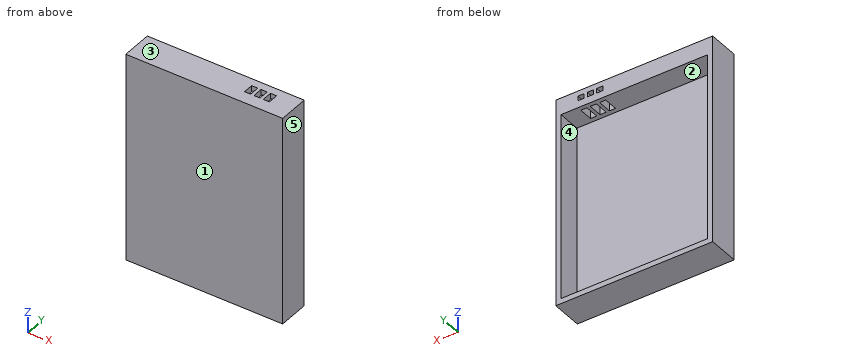
Autodesk Inventor part; units mm, degrees
ref_plane "YZ Plane" through (0, 0, 0) normal (1, 0, 0) x (0, 1, 0)
ref_plane "XZ Plane" through (0, 0, 0) normal (0, 1, 0) x (-1, 0, 0)
ref_plane "XY Plane" through (0, 0, 0) normal (0, 0, 1) x (1, 0, 0)
sketch "Sketch2" plane through (0, 0, 0) normal (0, 1, 0) x (-1, 0, 0)
  line L0 (11.0925, -17.7456) -> (-22.3075, -17.7456)
  line L1 (-22.3075, -17.7456) -> (-22.3075, 24.2544)
  line L2 (-22.3075, 24.2544) -> (11.0925, 24.2544)
  line L3 (11.0925, 24.2544) -> (11.0925, -17.7456)
  point P0 (0, 0)
  dimension "d2" = 42
  dimension "d3" = 33.4
extrude "Extrusion1" add sketch "Sketch2" along normal blind 6
sketch "Sketch3" plane through (0, 6, 0) normal (0, 1, 0) x (1, 0, 0)
  line L0 (-9.9925, 16.6456) -> (21.2075, 16.6456)
  line L1 (21.2075, 16.6456) -> (21.2075, -23.1544)
  line L2 (21.2075, -23.1544) -> (-9.9925, -23.1544)
  line L3 (-9.9925, -23.1544) -> (-9.9925, 16.6456)
  line L4 (22.3075, 17.7456) -> (-11.0925, 17.7456)
  line L5 (-11.0925, 17.7456) -> (-11.0925, -24.2544)
  line L6 (22.3075, -24.2544) -> (22.3075, 17.7456)
  line L7 (-11.0925, -24.2544) -> (22.3075, -24.2544)
  point P0 (0, 0)
  dimension "d6" = 1.1
  dimension "d7" = 1.1
  dimension "d8" = 1.1
  dimension "d9" = 1.1
  dimension "d10" = 39.8
extrude "Extrusion2" cut sketch "Sketch3" against normal blind 4.9 contours L0 L1 L2 L3
sketch "Sketch4" plane through (0, 0, 0) normal (0, -1, 0) x (1, 0, 0)
  line L0 (22.3075, -17.7456) -> (-11.0925, -17.7456)
  line L1 (-11.0925, -17.7456) -> (-11.0925, 24.2544)
  line L2 (22.3075, -17.7456) -> (-11.0925, -17.7456)
  line L3 (-11.0925, -17.7456) -> (-11.0925, 24.2544)
  line L4 (-11.0925, 24.2544) -> (22.3075, 24.2544)
  line L5 (22.3075, 24.2544) -> (22.3075, -17.7456)
  point P0 (0, 0)
extrude "Extrusion3" add sketch "Sketch4" along normal blind 0.6
sketch "Sketch5" plane through (-11.0925, 6, 24.2544) normal (0, 0, 1) x (1, 0, 0)
  line L0 (33.4, -6.6) -> (33.4, 0)
  line L1 (33.4, -6.6) -> (0, -6.6)
  line L2 (0, -6.6) -> (0, -2.5)
  line L3 (0, -2.5) -> (33.4, -2.5)
  line L4 (33.4, -2.5) -> (33.4, -6.6)
  point P0 (11.0925, -6)
  point P1 (33.4, -2.5)
extrude "Extrusion4" add sketch "Sketch5" along normal blind 3
sketch "Sketch6" plane through (21.2075, 6, 23.1544) normal (0, 0, -1) x (-1, 0, 0)
  line L0 (3.6, -0.9) -> (4.9, -0.9)
  line L1 (4.9, -0.9) -> (4.9, -3.9)
  line L2 (4.9, -3.9) -> (3.6, -3.9)
  line L3 (3.6, -3.9) -> (3.6, -0.9)
  line L4 (0, -4.9) -> (31.2, -4.9)
  line L5 (5.6, -0.9) -> (6.9, -0.9)
  line L6 (6.9, -0.9) -> (6.9, -3.9)
  line L7 (6.9, -3.9) -> (5.6, -3.9)
  line L8 (5.6, -3.9) -> (5.6, -0.9)
  line L9 (7.6, -0.9) -> (8.9, -0.9)
  line L10 (8.9, -0.9) -> (8.9, -3.9)
  line L11 (8.9, -3.9) -> (7.6, -3.9)
  line L12 (7.6, -3.9) -> (7.6, -0.9)
  point P0 (21.2075, -6)
  point P1 (0, 0)
  dimension "d17" = 3
  dimension "d18" = 1.3
  dimension "d19" = 3.6
  dimension "d20" = 1
  dimension "d23" = 3
  dimension "d24" = 1.3
  dimension "d25" = 3
  dimension "d26" = 1.3
  dimension "d27" = 1
  dimension "d28" = 1
  dimension "d29" = 0.7
  dimension "d30" = 0.7
sketch "Sketch7" plane through (-11.0925, 3.5, 24.2544) normal (0, 1, 0) x (1, 0, 0)
  line L0 (0, 0) -> (33.4, 0)
  line L1 (0, 42) -> (0, -3)
  line L2 (33.4, 0) -> (0, 0)
  line L3 (0, 0) -> (0, -3)
  line L4 (0, -3) -> (33.4, -3)
  line L5 (33.4, -3) -> (33.4, 0)
  point P0 (11.0925, 24.2544)
extrude "Extrusion5" add sketch "Sketch7" along normal blind 2.5
extrude "Extrusion6" cut sketch "Sketch6" against normal through all
sketch "Sketch8" plane through (0, 6, 0) normal (0, 1, 0) x (1, 0, 0)
  point P0 (0, 0)
sketch "Sketch9" plane through (16.3075, 2.1, 23.1544) normal (0, 1, 0) x (1, 0, 0)
  line L0 (1.3, 0) -> (1.3, -4.1)
  line L1 (0, 0) -> (0, -4.1)
  line L2 (1.3, -2.3) -> (0, -2.3)
  line L3 (0, -2.3) -> (0, -2)
  line L4 (0, -2) -> (1.3, -2)
  line L5 (1.3, -2) -> (1.3, -2.3)
  line L6 (0, 0) -> (1.3, 0)
  line L7 (-0.7, -2.3111) -> (-2, -2.3111)
  line L8 (-2, -2.3111) -> (-2, -2.0111)
  line L9 (-2, -2.0111) -> (-0.7, -2.0111)
  line L10 (-0.7, -2.0111) -> (-0.7, -2.3111)
  line L11 (-0.7, 0) -> (-0.7, -4.1)
  line L12 (-2, 0) -> (-0.7, 0)
  line L13 (-2.7, -2.3) -> (-4, -2.3)
  line L14 (-4, -2) -> (-2.7, -2)
  line L15 (-2.7, -2) -> (-2.7, -2.3)
  line L16 (-4, -2.3) -> (-4, -2)
  line L17 (-4, 0) -> (-2.7, 0)
  point P0 (-16.3075, 23.1544)
  point P1 (1.3, -2)
  point P2 (0, -2.3)
  dimension "d33" = 0.3
  dimension "d34" = 2
  dimension "d35" = 0.3
  dimension "d36" = 1.3
  dimension "d37" = 0
  dimension "d38" = 2.0111
  dimension "d39" = 0.3
  dimension "d40" = 1.3
  dimension "d41" = 0
  dimension "d42" = 2
extrude "Extrusion7" add sketch "Sketch9" along normal up to surface (3.9 mm away) contours L0 L2 L1 L4 | L7 L8 L9 L10 | L13 L16 L14 L15
sketch "Sketch10" plane through (0, 6, 0) normal (0, 1, 0) x (1, 0, 0)
  line L0 (17.6075, -25.6544) -> (16.3075, -25.6544)
  line L1 (16.3075, -25.6544) -> (16.3075, -24.6544)
  line L2 (16.3075, -24.6544) -> (17.6075, -24.6544)
  line L3 (17.6075, -24.6544) -> (17.6075, -25.6544)
  line L4 (21.2075, -23.1544) -> (-9.9925, -23.1544)
  line L5 (13.6075, -25.6544) -> (12.3075, -25.6544)
  line L6 (12.3075, -25.6544) -> (12.3075, -24.6544)
  line L7 (12.3075, -24.6544) -> (13.6075, -24.6544)
  line L8 (13.6075, -24.6544) -> (13.6075, -25.6544)
  line L9 (15.6075, -25.6544) -> (14.3075, -25.6544)
  line L10 (14.3075, -25.6544) -> (14.3075, -24.6544)
  line L11 (14.3075, -24.6544) -> (15.6075, -24.6544)
  line L12 (15.6075, -24.6544) -> (15.6075, -25.6544)
  line L13 (13.6075, -25.4544) -> (13.6075, -27.2544)
  point P0 (0, 0)
  point P1 (17.6075, -23.1544)
  point P2 (15.6075, -27.2544)
  dimension "d45" = 1.3
  dimension "d46" = 1
  dimension "d47" = 0
  dimension "d48" = 1.5
  dimension "d49" = 1.3
  dimension "d50" = 1
  dimension "d51" = 1.3
  dimension "d52" = 1
  dimension "d53" = 1.5
  dimension "d54" = 1.5
  dimension "d55" = 0
  dimension "d56" = 0
extrude "Extrusion8" cut sketch "Sketch10" against normal blind 1.5
sketch "Sketch11" plane through (-11.0925, 6, 27.2544) normal (0, 0, 1) x (1, 0, 0)
  line L0 (28.7, 0) -> (28.7, -0.9)
  line L1 (27.4, -3.9) -> (27.4, -0.9)
  line L2 (28.7, -0.9) -> (27.4, -0.9)
  line L3 (27.4, -0.9) -> (27.4, -1.7)
  line L4 (27.4, -1.7) -> (28.7, -1.7)
  line L5 (28.7, -1.7) -> (28.7, -0.9)
  line L6 (26.7, 0) -> (26.7, -0.9)
  line L7 (25.4, -3.9) -> (25.4, -1.5)
  line L8 (26.7, -0.9) -> (25.4, -0.9)
  line L9 (25.4, -0.9) -> (25.4, -1.7)
  line L10 (25.4, -1.7) -> (26.7, -1.7)
  line L11 (26.7, -1.7) -> (26.7, -0.9)
  line L12 (24.7, -0.9) -> (24.7, -3.9)
  line L13 (23.4, -3.9) -> (23.4, -0.9)
  line L14 (24.7, -0.9) -> (23.4, -0.9)
  line L15 (23.4, -0.9) -> (23.4, -1.7)
  line L16 (23.4, -1.7) -> (24.7, -1.7)
  line L17 (24.7, -1.7) -> (24.7, -0.9)
  point P0 (11.0925, -6)
  point P1 (24.7, -1.7)
  dimension "d59" = 0.8
extrude "Extrusion9" add sketch "Sketch11" against normal up to surface (1.6 mm away)
sketch "Sketch12" plane through (0, 6, 0) normal (0, 1, 0) x (1, 0, 0)
  line L0 (-11.0925, -27.2544) -> (22.3075, -27.2544)
  line L1 (-11.0925, 17.7456) -> (-11.0925, -27.2544)
  line L2 (22.3075, -27.2544) -> (-11.0925, -27.2544)
  line L3 (-11.0925, -27.2544) -> (-11.0925, -26.7544)
  line L4 (-11.0925, -26.7544) -> (22.3075, -26.7544)
  line L5 (22.3075, -26.7544) -> (22.3075, -27.2544)
  line L6 (17.6075, -25.6544) -> (16.3075, -25.6544)
  point P0 (0, 0)
  dimension "d62" = 1.1
extrude "Extrusion10" cut sketch "Sketch12" against normal through all
properties part number "battery-holder"
Can you work these out from the model? Positions are in its coordinate system, mm. Face numbers are marked on the shaded views. A direction names the side the tool comes from. Round coordinates to 2 decimals unless told otherwise and drop trailing zeros. Loops run counter-clockwise (first coordinate to the right, second up) from the corner with the lowest first, then second, coordinate; pieces in that order, holes last. Notation, with made-up numbers: M -30,76 L -18,76 A17 cw -18,92 Z; hole C 43.5,-1.75 d11. An arc over 180 degrees is marked long. Answer as a JSON object with one key per item and string values. Group by question number.
Q1. Imagine slicing it at C-C, the plane z = 10. Please give me the cut outline in (x, y), then the cut area to 3 significant figures.
Q2. Please list where these lines run through material, in increasing order: L1, parallel to X at y = 1.25, z = -11; L2, parallel to Z at x = 19.5, y = 1.5; L3, parallel to Z at x = 14.5, y = 4.
Q3. Will this pin go through, and if not, where does the flat tip stop? pin 1 (4 mm diameter, centred on x = -2, z = 13, fed in from +Y).
Q4. We'd pull the mould along Z, two halves only. Please class the marked faces 3, 4 and 5: +Z half, -Z half, draft (parallel to the pull), parting line (faces both ways), or undercut.
Q5. Imagine slicing it at A-A, the plane x = 15. Please give me the cut outline in (y, z), then the cut area to 3 significant figures.
Q6. On a 3-axis mill with a long thin cutter (end or side, diameter ignored), from which of +Z, -Z, +X, -X, +Y, -Y can I reach the whole of each face in a straight line? I mean the marked faces 1 and 2. Say none if no direction works.
Q7. Imagine slicing it at D-D, the plane x = 4. Please give me the cut outline in (y, z).
Findings:
{
 "1": {"outline": "M -11.09,-0.6 L 22.31,-0.6 L 22.31,6 L 21.21,6 L 21.21,1.1 L -9.99,1.1 L -9.99,6 L -11.09,6 Z", "area": "67.6 mm2"},
 "2": {"L1": "x = -11.09 to -9.99, 21.21 to 22.31", "L2": "z = -17.75 to -16.65, 23.15 to 26.75", "L3": "z = -17.75 to -16.65, 25.17 to 25.47"},
 "3": {"pin 1": "stops at y = 1.1"},
 "4": {"face 3": "+Z half", "face 4": "undercut", "face 5": "draft"},
 "5": {"outline": "M -0.6,-17.75 L 6,-17.75 L 6,-16.65 L 1.1,-16.65 L 1.1,23.15 L 2.1,23.15 L 2.1,25.17 L 4.5,25.17 L 4.5,25.47 L 2.1,25.47 L 2.1,26.75 L -0.6,26.75 Z; M 4.3,25.65 L 6,25.65 L 6,26.75 L 4.3,26.75 Z; M 5.1,23.15 L 6,23.15 L 6,24.65 L 5.1,24.65 Z", "area": "88.6 mm2"},
 "6": {"face 1": "+Z, -Z, +X, -X, -Y", "face 2": "+Y"},
 "7": {"outline": "M -0.6,-17.75 L 6,-17.75 L 6,-16.65 L 1.1,-16.65 L 1.1,23.15 L 6,23.15 L 6,26.75 L -0.6,26.75 Z"}
}
